Can you work these out from the model? Positions are in its coordinate system, mm. Coordinates: 2 decimals unless noted, no trailing zeros. Order: outer loops, then holes, each group sorted by start corner. A loop starts at its lowest first (then second) coordinate and runs counter-clockwise, first axis right, second up. Notation, with made-up numbers: (41, 87.25) -> (70, 87.25) arc R31 cw to (70, 118.25) -> close; hole circle Ø10 at (12.25, 63). An arc over 180 degrees is marked (long way). Write item = value, one per line.
```python
from build123d import *

# Parameters (mm, degrees)
BOSS_EXTRUDE1_DEPTH = 2
BOSS_EXTRUDE2_START = -3
SKETCH1_3_R         = 2.75
BOSS_EXTRUDE2_DEPTH = 3


with BuildPart() as part:
    # Sketch1 → Boss-Extrude1 (new body)
    with BuildSketch(Plane(origin=(0, 0, 0), x_dir=(1, 0, 0), z_dir=(0, 1, 0))):
        with BuildLine():
            Line((37, 2.75), (0, 2.75))
            ThreePointArc((0, 2.75), (-2.75, 0), (0, -2.75))
            Line((0, -2.75), (37, -2.75))
            Line((37, -2.75), (37, 2.75))
        make_face()
    extrude(amount=BOSS_EXTRUDE1_DEPTH)

    # Sketch1_3 → Boss-Extrude2 (add)
    with BuildSketch(Plane(origin=(0, 0, 0), x_dir=(1, 0, 0), z_dir=(0, 1, 0)).offset(BOSS_EXTRUDE2_START)):
        with Locations(Location((12, 0, 0), (0, 0, 270))):
            Circle(SKETCH1_3_R)
        with Locations(Location((0, 0, 0), (0, 0, 270))):
            Circle(SKETCH1_3_R)
    extrude(amount=BOSS_EXTRUDE2_DEPTH)


solid = part.part
```
Item 1: If we mould it in two halves opening along X, with no side actions, what happens to faces 1 (the flat face through (17, 2, 0)), 2 (the flat face through (37, 1, 0)), 3 (the cylindrical face through (14.727, -1.521, -0.358))? For each: pulls with the +X half, pulls with the -X half, needs draft (parallel to the pull), parting line crosses it, or undercut.
A:
face_1 = needs draft
face_2 = pulls with the +X half
face_3 = undercut
Item 2: I want a section at A-A, the plane z = 0. Please give me the cut outline in (x, y).
A:
outline = (-2.75, -3) -> (2.75, -3) -> (2.75, 0) -> (9.25, 0) -> (9.25, -3) -> (14.75, -3) -> (14.75, 0) -> (37, 0) -> (37, 2) -> (-2.75, 2) -> close
Item 3: I want a section at C-C, the plane x = 34. Please give me the cut outline in (y, z), plus the area to 3 significant figures.
A:
outline = (0, -2.75) -> (2, -2.75) -> (2, 2.75) -> (0, 2.75) -> close
area = 11.0 mm2
Item 4: If I drill on probe 1 along Y at (x, z) = (33.5, 2.4); probe 2 along X at (y, z) = (-1.1, 0.6); probe 3 along X at (y, z) = (-2.2, 0.8), over which ranges is the centre line in solid material (lowest first)?
A:
probe_1 = 0 to 2
probe_2 = -2.68 to 2.68, 9.32 to 14.68
probe_3 = -2.63 to 2.63, 9.37 to 14.63
Item 5: I'm going to push flat-ended pins straight in: P1, Ø3, axis at y = 0.5, z = 1.5, coming from the -X side; P2, Ø3, axis at x = 6, z = 1, coming from the -Y side. Where does each tip first touch, or does it pass through?
A:
P1 = -2.75
P2 = 0
Item 6: I want a section at D-D, the plane z = 1.7. Please give me the cut outline in (x, y).
A:
outline = (-2.16, -3) -> (2.16, -3) -> (2.16, 0) -> (9.84, 0) -> (9.84, -3) -> (14.16, -3) -> (14.16, 0) -> (37, 0) -> (37, 2) -> (-2.16, 2) -> close
Item 7: I want a section at B-B, the plane y = -1.35. Please give me the cut outline in (x, z).
A:
outline = circle Ø5.5 at (0, 0); circle Ø5.5 at (12, 0)
